```python
from build123d import *

# Parameters (mm, degrees)
SKETCH1_R           = 1.70053
BOSS_EXTRUDE1_DEPTH = 6.35
FILLET1_R           = 2.54


with BuildPart() as part:
    # Sketch1 → Boss-Extrude1 (new body)
    with BuildSketch(Plane(origin=(0, 0, 0), x_dir=(1, 0, 0), z_dir=(0, 1, 0))):
        Polygon((125.453583476, -114.442232973), (145.604758319, -98.979692676), (139.806305708, -91.42300211), (127.211821431, -101.087089795), (117.161170238, -87.988826147), (109.604479672, -93.787278758), align=None)
        with Locations(Location((117.248460029, -95.925846163, 0), (0, 0, 270))):
            Circle(SKETCH1_R, mode=Mode.SUBTRACT)
        with Locations(Location((137.667738303, -99.066982467, 0), (0, 0, 270))):
            Circle(SKETCH1_R, mode=Mode.SUBTRACT)
    extrude(amount=BOSS_EXTRUDE1_DEPTH)

    # Fillet1
    fillet1_edges = [part.edges().sort_by_distance(p)[0] for p in [
        (139.806305708, 3.175, 91.42300211),
        (145.604758319, 3.175, 98.979692676),
        (125.453583476, 3.175, 114.442232973),
        (109.604479672, 3.175, 93.787278758),
        (117.161170238, 3.175, 87.988826147),
    ]]
    fillet(fillet1_edges, radius=FILLET1_R)


solid = part.part
```
Could you check a few things on this model? Use its own coordinates, in mm. A direction names the side the tool comes from. Give positions to 0.01 mm unless a question says otherwise; leave off trailing zeros. Write each loop counter-clockwise with the first axis right and the second up, starting at its lowest first coordinate (ties: lowest second). Pieces come first, ordered by that corner, then holes. Notation, with made-up numbers: (-21.5, 71.5) - (26.5, 71.5) arc R18 cw to (26.5, 83.5) - close; hole circle Ø11 at (31, 59.5). An arc over 180 degrees is marked (long way). One line per item, written item: value. Start each with the question number.
Item 1: Please list where these lines run through material, in increasing order: line 1 (X direction, y = 2, z = 95.5); line 2 (X direction, y = 5.25, z = 97.75); line 3 (X direction, y = 1.5, z = 101) (3 decimals). Write a range as from..to.
Item 2: If we mould it in two halves opening along Z, with no side actions, what happens to faces 1 (the face through (144.558, 3.219, 98.87)), 2 (the face through (127, 6.35, 104)), 3 (the face through (117.323, 3.131, 94.227))? For each: +Z half, -Z half, draft (parallel to the pull), parting line (faces both ways), or undercut.
Item 3: Imagine slicing it at C-C, the plane z = 111.5. List the corners of the cut face in (x, y) for me, and give its area (3 significant figures).
Item 4: Imagine slicing it at B-B, the plane x = 116. List the corners of the cut face in (y, z) for me, and give its area (3 significant figures).
Item 5: I'm going to push flat-ended pins straight in: pin 1 (2 mm diameter, centred on y = 5, z = 107, fed in from -X); pin 2 (1 mm diameter, centred on x = 124.5, y = 5, fed in from +Z). Where does each tip first touch, or does it pass through?
Item 6: Which directions (+Z, -Z, +X, -X, +Y, -Y) give clear straight access to the entire face, cutting with the end or side of a thin tool? Please do faces 4 (the face through (132.58, 3.13, 96.97)), 5 (the face through (117.44, 3.13, 104)).
Item 7: Imagine slicing it at A-A, the plane y = 5. List the corners of the cut face in (x, z) for me.
Item 8: Imagine slicing it at D-D, the plane x = 123.5. List the corners of the cut face in (y, z) for me.
Geometry says:
1. line 1: 110.95..115.6, 118.89..122.92, 134.49..142.93
1. line 2: 112.65..124.65, 131.56..136.59, 138.74..144.47
1. line 3: 115.139..127.145, 127.325..142.972
2. face 1: parting line
2. face 2: draft
2. face 3: undercut
3. outline: (123.2, 0) - (129.29, 0) - (129.29, 6.35) - (123.2, 6.35) - close
3. area: 38.7 mm^2
4. outline: (0, 89.11) - (6.35, 89.11) - (6.35, 94.77) - (0, 94.77) - close; (0, 97.08) - (6.35, 97.08) - (6.35, 102.12) - (0, 102.12) - close
4. area: 68.0 mm^2
5. pin 1: x = 118.98
5. pin 2: z = 113.25
6. face 4: -Z, +Y, -Y
6. face 5: +Z, -X, +Y, -Y
7. outline: (111.15, 95.8) arc R2.54 ccw to (111.62, 92.24) - (115.15, 89.54) arc R2.54 ccw to (118.71, 90) - (127.21, 101.09) - (137.79, 92.97) arc R2.54 ccw to (141.35, 93.44) - (144.06, 96.96) arc R2.54 ccw to (143.59, 100.53) - (127.47, 112.9) arc R2.54 ccw to (123.91, 112.43) - close; hole circle Ø3.4 at (117.25, 95.93); hole circle Ø3.4 at (137.67, 99.07)
8. outline: (0, 96.25) - (6.35, 96.25) - (6.35, 111.9) - (0, 111.9) - close
